The listing builds one solid part. Answer for the finished solid, in the listing's coordinates (mm). Face numbers are marked on the shaded views. Coordinates: 2 decimals unless noted, no trailing zeros. Order: outer loops, then holes, each group sorted by start corner. A loop starts at its lowest first (then second) coordinate and runs counter-clockwise, first axis right, second up. Notation, with made-up numbers: (-17, 9.25) -> (-6, 9.25) arc R29 cw to (-6, 39.25) -> close; hole circle Ø10 at (24.25, 74). An arc over 180 degrees is marked (long way). Write each question's results on one line, items separated by ' | '. Start each with the question number.
(1) The part is cut by section C-C, the plane x = -1.25. Give the vertices of the cut face in (y, z).
(2) Determine the mould class of the marked faces 1, 2 and 3 for opening direction Z: +Z half, -Z half, draft (parallel to the pull), parting line (faces both ways), or undercut.
(3) Given pin 1 (25 mm diameter, centred on y = 0, z = 0, fed in from -X); pin 2 (5 mm diameter, centred on x = 5, z = 9, fed in from -Y); pin 3 (6 mm diameter, centred on x = 3, z = -13.5, fed in from +Y), each flat-ended and moving along its own axis, determine where each tip first touches the part or whether it passes through.
(4) Straight lines are drawn through the part: L1, parallel to X at y = 17, z = -3.5; L2, parallel to Y at x = -0.8, z = 0; L3, parallel to Z at x = -3.25, y = -4.5. For each, find the intervals that lie inside material, in ascending order.
```python
from build123d import *

# Parameters (mm, degrees)
CHAMFER1_SIZE = 2
FILLET1_R     = 1.5


with BuildPart() as part:
    # Sketch1 → Revolve1 (revolve)
    with BuildSketch(Plane.XY, mode=Mode.PRIVATE) as revolve1_sk:
        Polygon((-7, 14), (-7, 25.75), (7, 25.75), (7, 14), (7, 7), (4, 7), (4, 14), (4, 21), (-4, 21), (-4, 14), align=None)
    revolve(revolve1_sk.sketch.rotate(Axis((0, 0, 0), (-1, 0, 0)), 90), axis=Axis((0, 0, 0), (-1, 0, 0)))

    # Chamfer1
    chamfer1_edges = [part.edges().sort_by_distance(p)[0] for p in [
        (7, 0, 25.75),
        (-7, 0, 25.75),
        (-4, 0, 21),
        (4, 0, 21),
    ]]
    chamfer(chamfer1_edges, length=CHAMFER1_SIZE)

    # Fillet1
    fillet1_edges = [part.edges().sort_by_distance(p)[0] for p in [
        (7, 0, 7),
        (-7, 0, 14),
        (-4, 0, 14),
        (4, 0, 7),
    ]]
    fillet(fillet1_edges, radius=FILLET1_R - 0.0001)  # a hair under: the kernel refuses the full size


solid = part.part
```
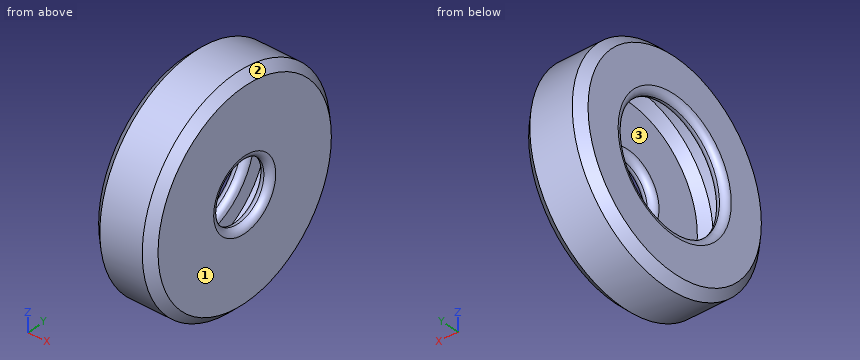
Established:
1) outline: circle Ø51.5 at (0, 0); hole circle Ø42 at (0, 0)
2) face 1: draft | face 2: parting line | face 3: undercut
3) pin 1: stops at x = 4 | pin 2: stops at y = -24.92 | pin 3: stops at y = 23.51
4) L1: x = -7 to -4, 4 to 7 | L2: y = -25.75 to -21, 21 to 25.75 | L3: z = -25.35 to -19.23, 19.23 to 25.35
